Autodesk Inventor part; units mm, degrees
ref_plane "YZ Plane" through (0, 0, 0) normal (1, 0, 0) x (0, 1, 0)
ref_plane "XZ Plane" through (0, 0, 0) normal (0, 1, 0) x (-1, 0, 0)
ref_plane "XY Plane" through (0, 0, 0) normal (0, 0, 1) x (1, 0, 0)
sketch "Sketch1" plane through (0, 0, 0) normal (0, 1, 0) x (-1, 0, 0)
  line L0 (0, 0) -> (30.1625, 0)
  line L1 (30.1625, 0) -> (30.1625, -106.3625)
  line L2 (30.1625, -106.3625) -> (0, -106.3625)
  line L3 (0, -106.3625) -> (0, 0)
  dimension "d0" = 30.1625
  dimension "d1" = 106.3625
extrude "Extrusion1" add sketch "Sketch1" along normal blind 9.525
sketch "Sketch2" plane through (0, 0, 0) normal (1, 0, 0) x (0, 0, -1)
  line L0 (0, 0) -> (0, 9.525) construction
  line L1 (0, 9.525) -> (106.3625, 9.525) construction
  line L2 (106.3625, 0) -> (106.3625, 9.525) construction
  line L3 (28.575, 9.525) -> (106.3625, 9.525) construction
  line L4 (106.3625, 9.525) -> (106.3625, 0) construction
  line L5 (106.3625, 0) -> (28.575, 0) construction
  line L6 (28.575, 0) -> (28.575, 9.525) construction
  line L7 (28.575, 4.7625) -> (28.575, 0) construction
  line L8 (28.575, 4.7625) -> (28.575, 2.3813) construction
  line L9 (28.575, 2.3813) -> (33.655, 2.3813) construction
  line L10 (33.655, 2.3813) -> (46.355, 2.3813)
  line L11 (46.355, 2.3813) -> (46.355, 7.1437)
  line L12 (46.355, 7.1437) -> (33.655, 7.1438)
  line L13 (33.655, 7.1438) -> (33.655, 2.3813)
  line L14 (46.355, 2.3813) -> (51.435, 2.3813) construction
  line L15 (51.435, 2.3813) -> (64.135, 2.3813)
  line L16 (64.135, 2.3813) -> (64.135, 7.1437)
  line L17 (64.135, 7.1437) -> (51.435, 7.1437)
  line L18 (51.435, 7.1437) -> (51.435, 2.3813)
  line L19 (64.135, 2.3813) -> (69.215, 2.3813)
  line L20 (69.215, 2.3813) -> (81.915, 2.3813)
  line L21 (81.915, 2.3813) -> (81.915, 7.1437)
  line L22 (81.915, 7.1437) -> (69.215, 7.1437)
  line L23 (69.215, 7.1437) -> (69.215, 2.3813)
  line L24 (81.915, 2.3813) -> (86.995, 2.3813)
  line L25 (81.915, 7.1437) -> (81.915, 2.3813)
  line L26 (86.995, 2.3813) -> (99.695, 2.3813)
  line L27 (99.695, 2.3813) -> (99.695, 7.1437)
  line L28 (99.695, 7.1437) -> (86.995, 7.1437)
  line L29 (86.995, 7.1437) -> (86.995, 2.3813)
  dimension "d7" = 2.3813
  dimension "d9" = 12.7
  dimension "d10" = 4.7625
  dimension "d12" = 12.7
  dimension "d13" = 4.7625
  dimension "d15" = 12.7
  dimension "d16" = 4.7625
  dimension "d20" = 28.575
  dimension "d21" = 12.7
  dimension "d22" = 4.7625
  dimension "d23" = 5.08
  dimension "d24" = 5.08
  dimension "d25" = 5.08
  dimension "d26" = 5.08
extrude "Extrusion2" cut sketch "Sketch2" against normal blind 9.525
fillet "Fillet1" radius 3.175 4 edges at (0, 4.7625, 0) (-30.1625, 4.7625, 0) (-30.1625, 4.7625, -106.3625) (0, 4.7625, -106.3625)
sketch "Sketch3" plane through (-26.9875, 0, 0) normal (0, 0, 1) x (1, 0, 0)
  line L0 (0, 0) -> (23.8125, 0) construction
  line L1 (11.9062, 0) -> (11.9062, 9.525) construction
  line L2 (23.8125, 9.525) -> (0, 9.525) construction
  circle A0 centre (11.9062, 4.7625) radius 2.54
  point P0 (26.9875, 0)
  dimension "d30" = 5.08
extrude "Extrusion3" add sketch "Sketch3" along normal blind 9.525
sketch "Sketch4" plane through (-9.525, 0, 0) normal (1, 0, 0) x (0, 0, -1)
  line L0 (33.655, 2.3813) -> (33.655, 7.1438) construction
  line L1 (33.655, 4.7625) -> (99.695, 4.7625) construction
  line L2 (99.695, 7.1437) -> (99.695, 2.3813) construction
  line L3 (40.005, 4.7625) -> (34.925, 4.7625) construction
  line L4 (34.925, 4.7625) -> (34.925, 6.0325) construction
  line L5 (34.925, 6.0325) -> (40.005, 6.0325) construction
  line L6 (40.005, 6.0325) -> (40.005, 4.7625) construction
  line L7 (57.785, 4.7625) -> (52.705, 4.7625) construction
  line L8 (52.705, 4.7625) -> (52.705, 6.0325) construction
  line L9 (52.705, 6.0325) -> (57.785, 6.0325) construction
  line L10 (57.785, 6.0325) -> (57.785, 4.7625) construction
  line L11 (75.565, 4.7625) -> (70.485, 4.7625) construction
  line L12 (70.485, 4.7625) -> (70.485, 6.0325) construction
  line L13 (70.485, 6.0325) -> (75.565, 6.0325) construction
  line L14 (75.565, 6.0325) -> (75.565, 4.7625) construction
  line L15 (93.345, 4.7625) -> (88.265, 4.7625) construction
  line L16 (88.265, 4.7625) -> (88.265, 6.0325) construction
  line L17 (88.265, 6.0325) -> (93.345, 6.0325) construction
  line L18 (93.345, 6.0325) -> (93.345, 4.7625) construction
  line L19 (93.345, 4.7625) -> (98.425, 4.7625) construction
  line L20 (75.565, 4.7625) -> (80.645, 4.7625) construction
  line L21 (57.785, 4.7625) -> (62.865, 4.7625) construction
  line L22 (40.005, 4.7625) -> (45.085, 4.7625) construction
  line L23 (34.925, 6.0325) -> (45.085, 6.0325)
  line L24 (45.085, 6.0325) -> (45.085, 4.7625)
  line L25 (45.085, 4.7625) -> (34.925, 4.7625)
  line L26 (34.925, 4.7625) -> (34.925, 6.0325)
  line L27 (52.705, 6.0325) -> (62.865, 6.0325)
  line L28 (62.865, 6.0325) -> (62.865, 4.7625)
  line L29 (62.865, 4.7625) -> (52.705, 4.7625)
  line L30 (52.705, 4.7625) -> (52.705, 6.0325)
  line L31 (70.485, 6.0325) -> (80.645, 6.0325)
  line L32 (80.645, 6.0325) -> (80.645, 4.7625)
  line L33 (80.645, 4.7625) -> (70.485, 4.7625)
  line L34 (70.485, 4.7625) -> (70.485, 6.0325)
  line L35 (88.265, 6.0325) -> (98.425, 6.0325)
  line L36 (98.425, 6.0325) -> (98.425, 4.7625)
  line L37 (98.425, 4.7625) -> (88.265, 4.7625)
  line L38 (88.265, 4.7625) -> (88.265, 6.0325)
  point P0 (0, 0)
  dimension "d33" = 5.08
  dimension "d34" = 1.27
  dimension "d35" = 5.08
  dimension "d36" = 1.27
  dimension "d37" = 5.08
  dimension "d38" = 1.27
  dimension "d39" = 5.08
  dimension "d40" = 1.27
  dimension "d41" = 5.08
  dimension "d42" = 5.08
  dimension "d43" = 5.08
  dimension "d44" = 5.08
extrude "Extrusion4" add sketch "Sketch4" along normal blind 6.35
properties part number "usbHub" material "ABS Plastic"
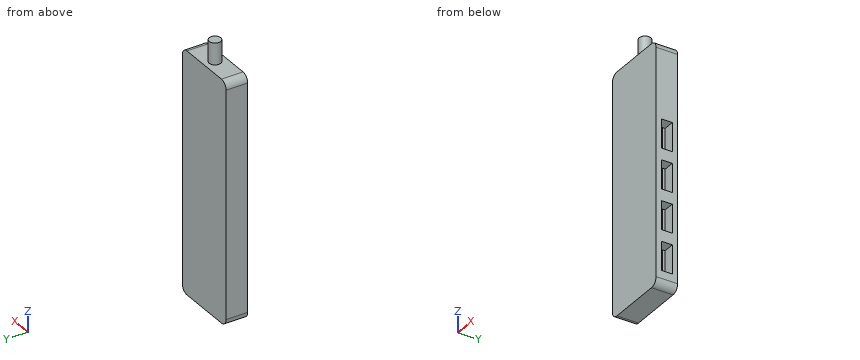
CAD build for the part. Positions are in the model's coordinates, mm. Round coordinates to 2 decimals unless told otherwise and drop trailing zeros. Write each loop counter-clockwise with the first axis right and the second up, starting at its lowest first coordinate (ties: lowest second). Pieces come first, ordered by that corner, then holes. Notation, with made-up numbers: M -5.75,27 L 32.25,27 A28 ccw 32.25,56 Z; hole C 16.5,-12.5 d9. An arc over 180 degrees is marked long. Put each result on its own line as item: value. Start each with the question number.
1) Saw through at B-B, the plane z = -43. Write the cut outline in (x, y) (1 decimal), and give its area (3 significant figures).
2) Pin check, flat tips, straight feed: pin 1 Ø1.4 at (y, z) = (5.5, -40) entering from +X (3 decimals); pin 2 Ø1.4 at (y, z) = (4, -41) entering from +X (3 decimals); pin 3 Ø0.6 at (x, y) = (-7.5, 5.5) entering from +Z. Stop position of each tip, or through.
3) Saw through at C-C, the plane x = -25.5. Write the cut outline in (y, z) (1 decimal).
4) Drill centre lines: probe 1 along Z at (x, y) = (-6, 6.75) (1 decimal); probe 2 along Y at (x, z) = (-8.5, -98) (1 decimal); probe 3 along Y at (x, z) = (-5, -63) (3 decimals). Where is each one in solid material? Low to high. Write a range as [from, to].
5) Saw through at A-A, the plane x = -6. Count the separate pieces of the cut face and the enclosed holes in it, and give its area (3 significant figures).
Resolved:
1. outline: M -30.2,0 L 0,0 L 0,2.4 L -9.5,2.4 L -9.5,4.8 L -3.2,4.8 L -3.2,6 L -9.5,6 L -9.5,7.1 L 0,7.1 L 0,9.5 L -30.2,9.5 Z
1. area: 250 mm²
2. pin 1: x = -3.175
2. pin 2: x = -9.525
2. pin 3: z = 0
3. outline: M 0,-106.4 L 9.5,-106.4 L 9.5,0 L 0,0 Z
4. probe 1: [-106.4, -99.7], [-87, -81.9], [-69.2, -64.1], [-51.4, -46.4], [-33.7, 0]
4. probe 2: [0, 2.4], [4.8, 6], [7.1, 9.5]
4. probe 3: [0, 2.381], [7.144, 9.525]
5. separate pieces: 5
5. enclosed holes: 4
5. area: 823 mm²
